from build123d import *

# Parameters (mm, degrees)
SKETCH_1_W               = 10
SKETCH_1_H               = 38
SKETCH_1_R               = 1.1
EXTRUDE_1_DEPTH          = 0.75
EXTRUDE_1_DEPTH_BACK     = 0.75
SKETCH_3_W               = 20
SKETCH_3_H               = 38.036879249
EXTRUDE_2_DEPTH          = 1.5
EXTRUDE_3_DEPTH          = 0.75
EXTRUDE_3_DEPTH_BACK     = 0.75
EXTRUDE_4_DEPTH          = 38
CUT_EXTRUDE_1_DEPTH      = 10
CUT_EXTRUDE_1_DEPTH_BACK = 20
SKETCH_10_W              = 112.497058814
SKETCH_10_H              = 20.543414641
CUT_EXTRUDE_4_DEPTH      = 0.2
CUT_EXTRUDE_4_DEPTH_BACK = 0.2
SKETCH_11_W              = 104.514605189
SKETCH_11_H              = 21.657747512
CUT_EXTRUDE_5_DEPTH      = 0.2
CUT_EXTRUDE_5_DEPTH_BACK = 0.2


with BuildPart() as part:
    # Sketch 1 → Extrude 1 (new body, two sides)
    with BuildSketch(Plane.XY) as extrude_1_sk:
        with Locations((-4.101832994, 0.735234216)):
            Rectangle(SKETCH_1_W, SKETCH_1_H)
        with Locations((-6.601832994, -15.764765784)):
            Circle(SKETCH_1_R, mode=Mode.SUBTRACT)
        with Locations((-6.578411405, 17.235234216)):
            Circle(SKETCH_1_R, mode=Mode.SUBTRACT)
    extrude(amount=EXTRUDE_1_DEPTH)
    extrude(extrude_1_sk.sketch, amount=-EXTRUDE_1_DEPTH_BACK)

    # Sketch 3 → Extrude 2 (add)
    with BuildSketch(Plane(origin=(-0.5, 0, 0), x_dir=(0, 0, -1), z_dir=(1, 0, 0))):
        with Locations((0, 0.716794592)):
            Rectangle(SKETCH_3_W, SKETCH_3_H)
    extrude(amount=EXTRUDE_2_DEPTH)

    # Sketch 4 → Extrude 3 (add, two sides)
    with BuildSketch(Plane.XY) as extrude_3_sk:
        with BuildLine():
            Line((1, 19.735234216), (1, -18.298860138))
            ThreePointArc((1, -18.298860138), (51.989546932, -13.993809638), (101, 0.718187039))
            ThreePointArc((101, 0.718187039), (51.989546932, 15.430183716), (1, 19.735234216))
        make_face()
    extrude(amount=EXTRUDE_3_DEPTH)
    extrude(extrude_3_sk.sketch, amount=-EXTRUDE_3_DEPTH_BACK)

    # Sketch 5 → Extrude 4 (add)
    with BuildSketch(Plane(origin=(0, 19.735234216, 0), x_dir=(1, 0, 0), z_dir=(0, 1, 0))):
        with BuildLine():
            Line((1, -9), (1, -10))
            ThreePointArc((1, -10), (51.064071237, -7.900139791), (101, -3.75))
            Line((101, -3.75), (101, -2.75))
            ThreePointArc((101, -2.75), (51.071468752, -7.018500027), (1, -9))
        make_face()
        with BuildLine():
            Line((101, 2.75), (101, 3.75))
            ThreePointArc((101, 3.75), (51.064071237, 7.900139791), (1, 10))
            Line((1, 10), (1, 9))
            ThreePointArc((1, 9), (51.071468752, 7.018500027), (101, 2.75))
        make_face()
    extrude(amount=-EXTRUDE_4_DEPTH)

    # Sketch 8 → Cut-Extrude 1 (cut, two sides)
    with BuildSketch(Plane.XY.offset(10)) as cut_extrude_1_sk:
        with BuildLine():
            Line((13.103688801, -18.23809131), (101, -18.264765784))
            Line((101, -18.264765784), (101, 0.718187039))
            ThreePointArc((101, 0.718187039), (57.921072507, -12.790381672), (13.103688801, -18.23809131))
        make_face()
        with BuildLine():
            ThreePointArc((13.103688801, 19.674465387), (57.921072507, 14.22675575), (101, 0.718187039))
            Line((101, 0.718187039), (101, 19.701139862))
            Line((101, 19.701139862), (13.103688801, 19.674465387))
        make_face()
    extrude(amount=CUT_EXTRUDE_1_DEPTH, mode=Mode.SUBTRACT)
    extrude(cut_extrude_1_sk.sketch, amount=-CUT_EXTRUDE_1_DEPTH_BACK, mode=Mode.SUBTRACT)

    # Sketch 10 → Cut-Extrude 4 (cut, two sides)
    with BuildSketch(Plane(origin=(0, 19.735234216, 0), x_dir=(1, 0, 0), z_dir=(0, 1, 0))) as cut_extrude_4_sk:
        with Locations((46.49437126, 0.271707321)):
            Rectangle(SKETCH_10_W, SKETCH_10_H)
    extrude(amount=CUT_EXTRUDE_4_DEPTH, mode=Mode.SUBTRACT)
    extrude(cut_extrude_4_sk.sketch, amount=-CUT_EXTRUDE_4_DEPTH_BACK, mode=Mode.SUBTRACT)

    # Sketch 11 → Cut-Extrude 5 (cut, two sides)
    with BuildSketch(Plane(origin=(0, -18.301645033, 0), x_dir=(-1, 0, 0), z_dir=(0, -1, 0))) as cut_extrude_5_sk:
        with Locations((-51.541283716, 0.828873756)):
            Rectangle(SKETCH_11_W, SKETCH_11_H)
    extrude(amount=CUT_EXTRUDE_5_DEPTH, mode=Mode.SUBTRACT)
    extrude(cut_extrude_5_sk.sketch, amount=-CUT_EXTRUDE_5_DEPTH_BACK, mode=Mode.SUBTRACT)


solid = part.part
The listing builds one solid part. Answer for the finished solid, in the listing's coordinates (mm). A direction names the side the tool comes from. Coordinates: 2 decimals unless noted, no trailing zeros. Loops run counter-clockwise (first coordinate to the right, second up) from the corner with the lowest first, then second, coordinate; pieces in that order, holes last. Notation, with made-up numbers: M 45.25,56.5 L 77.25,56.5 A18 cw 77.25,86.5 Z; hole C -6,-14.5 d2. An arc over 180 degrees is marked long. Answer in a Markdown table with one row per item.
1) Find section B-B (z = -5.75). Determine the outline of the cut face in (x, y).
Answers below:
| item | result |
|---|---|
| outline | M -0.5,-18.1 L 1,-18.1 L 1,19.54 L -0.5,19.54 Z; M 69,-10.13 A247.18 ccw 79.96,-6.96 L 79.96,8.4 A247.18 ccw 69,11.57 Z |
2) Find section C-C (y = 9.5). Determine the outline of the cut face in (x, z), then the cut area to 3 significant figures.
Answers below:
| item | result |
|---|---|
| outline | M -9.1,-0.75 L -0.5,-0.75 L -0.5,-10 L 1,-10 A1222.24 ccw 76.36,-6.06 L 76.36,-5.14 A1095.84 cw 1,-9 L 1,-0.75 L 76.36,-0.75 L 76.36,0.75 L 1,0.75 L 1,9 A1095.84 cw 76.36,5.14 L 76.36,6.06 A1222.24 ccw 1,10 L -0.5,10 L -0.5,0.75 L -9.1,0.75 Z |
| area | 293 mm^2 |
3) Find the intervals of material crossed by probe 1 along Z at (x, y) = (2, 12); probe 2 along Z at (x, y) = (14, -6.5); probe 3 along X at (y, z) = (-10.5, 4.5), in increasing order.
Answers below:
| item | result |
|---|---|
| probe 1 | -9.98 to -8.98, -0.75 to 0.75, 8.98 to 9.98 |
| probe 2 | -9.65 to -8.71, -0.75 to 0.75, 8.71 to 9.65 |
| probe 3 | -0.5 to 1 |
4) Find section A-A (x = 54). Determine the outline of the cut face in (y, z).
Answers below:
| item | result |
|---|---|
| outline | M -13.6,-7.71 L 15.04,-7.71 L 15.04,-6.83 L -13.6,-6.83 Z; M -13.6,-0.75 L 15.04,-0.75 L 15.04,0.75 L -13.6,0.75 Z; M -13.6,6.83 L 15.04,6.83 L 15.04,7.71 L -13.6,7.71 Z |
5) Find section D-D (x = 23). Determine the outline of the cut face in (y, z).
Answers below:
| item | result |
|---|---|
| outline | M -17.75,-9.33 L 19.18,-9.33 L 19.18,-8.41 L -17.75,-8.41 Z; M -17.75,-0.75 L 19.18,-0.75 L 19.18,0.75 L -17.75,0.75 Z; M -17.75,8.41 L 19.18,8.41 L 19.18,9.33 L -17.75,9.33 Z |
6) Determine the mould class of faces 5 (the flat face through (39, 1, -0.75)), 6 (the flat face through (5, 19.535, 0)), 7 (the cylindrical face through (-6.817, 16.161, -0.01)), 8 (the cylindrical face through (59.92, -12.35, -6.64)) for opening direction Y: released by +Y, released by -Y, zero draft, split by the parting line, or undercut.
Answers below:
| item | result |
|---|---|
| face 5 | zero draft |
| face 6 | released by +Y |
| face 7 | undercut |
| face 8 | released by -Y |
7) Which of the six approach directions +Z, -Z, +X, -X, +Y, -Y give full straight-line access (tool end or side, diameter ignored) to faces 1 (the flat face through (5, -18.102, 0)), 2 (the flat face through (-5, 1, 0.75)), 3 (the flat face through (1, 1, 5)), 4 (the flat face through (39, 1, 0.75))?
Answers below:
| item | result |
|---|---|
| face 1 | +Z, -Z, +X, -Y |
| face 2 | +Z, -X, +Y, -Y |
| face 3 | +Y, -Y |
| face 4 | +X, +Y, -Y |
8) Given pin 1 (5 mm diameter, centred on y = 1, z = 6, fed in from -X); pin 2 (8 mm diameter, centred on y = -12, z = -4, fed in from -X); pin 3 (6 mm diameter, centred on x = 14.5, y = -2, fed in from -Z); pin 4 (9.5 mm diameter, centred on x = -6.5, y = -3, fed in from +Z), each flat-ended and moving along its own axis, determine where each tip first touches the part or whether it passes through.
Answers below:
| item | result |
|---|---|
| pin 1 | x = -0.5 |
| pin 2 | x = -9.1 |
| pin 3 | z = -9.73 |
| pin 4 | z = 0.75 |
